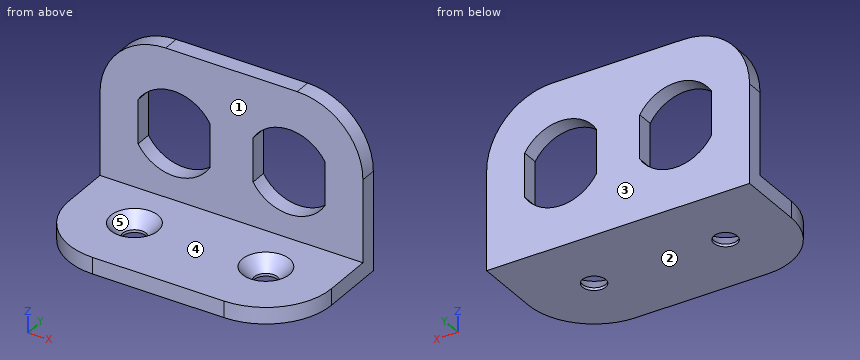
```python
from build123d import *

# Parameters (mm, degrees)
BOSS_EXTRUDE1_DEPTH                           = 50.8
CUT_EXTRUDE1_DEPTH                            = 66.068137364
FILLET1_R                                     = 12.7
CSK_FOR_8_FLAT_HEAD_SOCKET_CAP_SCREW1_A_COUNT = 2
CSK_FOR_8_FLAT_HEAD_SOCKET_CAP_SCREW1_A_PITCH = 25.4


with BuildPart() as part:
    # Sketch1 → Boss-Extrude1 (new body)
    with BuildSketch(Plane(origin=(0, 0, 0), x_dir=(0, 0, -1), z_dir=(1, 0, 0))):
        Polygon((0, 0), (-31.75, 0), (-31.75, -3.175), (-3.175, -3.175), (-3.175, -25.4), (0, -25.4), align=None)
    extrude(amount=BOSS_EXTRUDE1_DEPTH)

    # Sketch2 → Cut-Extrude1 (cut, through all)
    with BuildSketch(Plane(origin=(0, 0, 0), x_dir=(1, 0, 0), z_dir=(0, 1, 0))):
        with BuildLine():
            Line((7.3533, -11.634569083), (7.3533, -20.115430917))
            ThreePointArc((7.3533, -20.115430917), (14.2875, -24.003), (21.2217, -20.115430917))
            Line((21.2217, -20.115430917), (21.2217, -11.634569083))
            ThreePointArc((21.2217, -11.634569083), (14.2875, -7.747), (7.3533, -11.634569083))
        make_face()
        with BuildLine():
            Line((29.5783, -11.634569083), (29.5783, -20.115430917))
            ThreePointArc((29.5783, -20.115430917), (36.5125, -24.003), (43.4467, -20.115430917))
            Line((43.4467, -20.115430917), (43.4467, -11.634569083))
            ThreePointArc((43.4467, -11.634569083), (36.5125, -7.747), (29.5783, -11.634569083))
        make_face()
    extrude(amount=-CUT_EXTRUDE1_DEPTH, mode=Mode.SUBTRACT)

    # Fillet1
    fillet1_edges = [part.edges().sort_by_distance(p)[0] for p in [
        (50.8, -1.5875, 31.75),
        (50.8, -25.4, 1.5875),
        (0, -25.4, 1.5875),
        (0, -1.5875, 31.75),
    ]]
    fillet(fillet1_edges, radius=FILLET1_R)

    # Sketch4 → CSK for #8 Flat Head Socket Cap Screw1 (revolve, cut)
    with BuildSketch(Plane(origin=(12.7, -12.7, 3.175), x_dir=(0, -1, 0), z_dir=(1, 0, 0))):
        Polygon((0, 0), (0, 3.175), (2.2479, 3.175), (2.2479, 2.658961536), (4.5593, 0), align=None)
    csk_for_8_flat_head_socket_cap_screw1 = revolve(axis=Axis((12.7, -12.7, 9.525), (0, 0, -1)), mode=Mode.SUBTRACT)

    # CSK for #8 Flat Head Socket Cap Screw1 a: CSK for #8 Flat Head Socket Cap Screw1 ×2
    with Locations(*[(i * CSK_FOR_8_FLAT_HEAD_SOCKET_CAP_SCREW1_A_PITCH, 0, 0) for i in range(1, CSK_FOR_8_FLAT_HEAD_SOCKET_CAP_SCREW1_A_COUNT)]):
        add(csk_for_8_flat_head_socket_cap_screw1, mode=Mode.SUBTRACT)


solid = part.part
```
Check sheet for the modelled part. Datum: model origin and axes. Units: mm. Face numbers are marked on the shaded views. A direction names the side the tool comes from. Coordinates: 2 decimals unless noted, no trailing zeros. Order: outer loops, then holes, each group sorted by start corner. A loop starts at its lowest first (then second) coordinate and runs counter-clockwise, first axis right, second up. Notation, with made-up numbers: (-15.5, 37.25) -> (28.5, 37.25) arc R10 cw to (28.5, 55.25) -> close; hole circle Ø4 at (15.25, 87.5). An arc over 180 degrees is marked (long way). Write item = value, one per line. Start each with the question number.
1) Go/stop test with flat-tipped pins: P1, Ø6, axis at y = -14.5, z = 5.5, coming from the -X side; P2, Ø5, axis at y = -3, z = 27, coming from the +X side; P3, Ø5, axis at x = 33.5, y = -17, coming from the +Z side (3 decimals); P4, Ø8, axis at x = 6, z = 6.5, coming from the -Y side. Record where each tip stops, or that it passes through.
2) Cross-section at C-C (x = 6). Enter the section's corners in (y, z) (3 decimals), then the cut area to 3 significant figures.
3) Mould release check, pull along Y, two halves, no side actions. Record for the marked faces 3, 4 and 5: +Y half, -Y half, draft (parallel to the pull), parting line (faces both ways), or undercut.
4) Material ranges on L1, parallel to X at y = -12.7, z = 0.4; L2, parallel to Y at x = 38.1, z = 0.3; L3, parallel to Z at x = 17.5, y = -19.5 (3 decimals), recorded low to high.
5) Access from +Z, -Z, +X, -X, +Y, -Y to the whole of each face (thin tool, end or side, straight path). Record for the marked faces 1 and 2.
6) Cross-section at A-A (z = 12.5). Enter the section's corners in (x, y) (3 decimals).
7) Cross-section at B-B (y = -1.75). State how many separate pieces and enclosed holes the cut face has, then the cut area to 3 significant figures.
8) Cross-section at D-D (z = 4.5). Enter the section's corners in (x, y) (3 decimals), then the cut area to 3 significant figures.
Ans:
q1.P1 = 0
q1.P2 = 49.57
q1.P3 = 3.175
q1.P4 = -24.58
q2.outline = (-23.489, 0) -> (0, 0) -> (0, 29.839) -> (-3.175, 29.839) -> (-3.175, 3.175) -> (-23.489, 3.175) -> close
q2.area = 159 mm²
q3.face_3 = +Y half
q3.face_4 = draft
q3.face_5 = undercut
q4.L1 = 0 to 10.45, 14.95 to 35.85, 40.35 to 50.8
q4.L2 = -25.4 to -14.95, -10.45 to 0
q4.L3 = 0 to 3.175
q5.face_1 = +Z, +X, -X, -Y
q5.face_2 = -Z, +X, -X, +Y, -Y
q6.outline = (0, -3.175) -> (7.353, -3.175) -> (7.353, 0) -> (0, 0) -> close; (21.222, -3.175) -> (29.578, -3.175) -> (29.578, 0) -> (21.222, 0) -> close; (43.447, -3.175) -> (50.8, -3.175) -> (50.8, 0) -> (43.447, 0) -> close
q7.separate_pieces = 1
q7.enclosed_holes = 2
q7.area = 1,160 mm²
q8.outline = (0, -3.175) -> (50.8, -3.175) -> (50.8, 0) -> (0, 0) -> close
q8.area = 161 mm²
